Can you work these out from the drawing? Everything is in mm from the part's minimum corner. A direction names the side the tool comes from. Coordinates: 2 decimals unless noted, no trailing zeros. Loops run counter-clockwise (first coordinate to the right, second up) from the corner with the lowest first, then second, coordinate; pieces in that order, holes last.
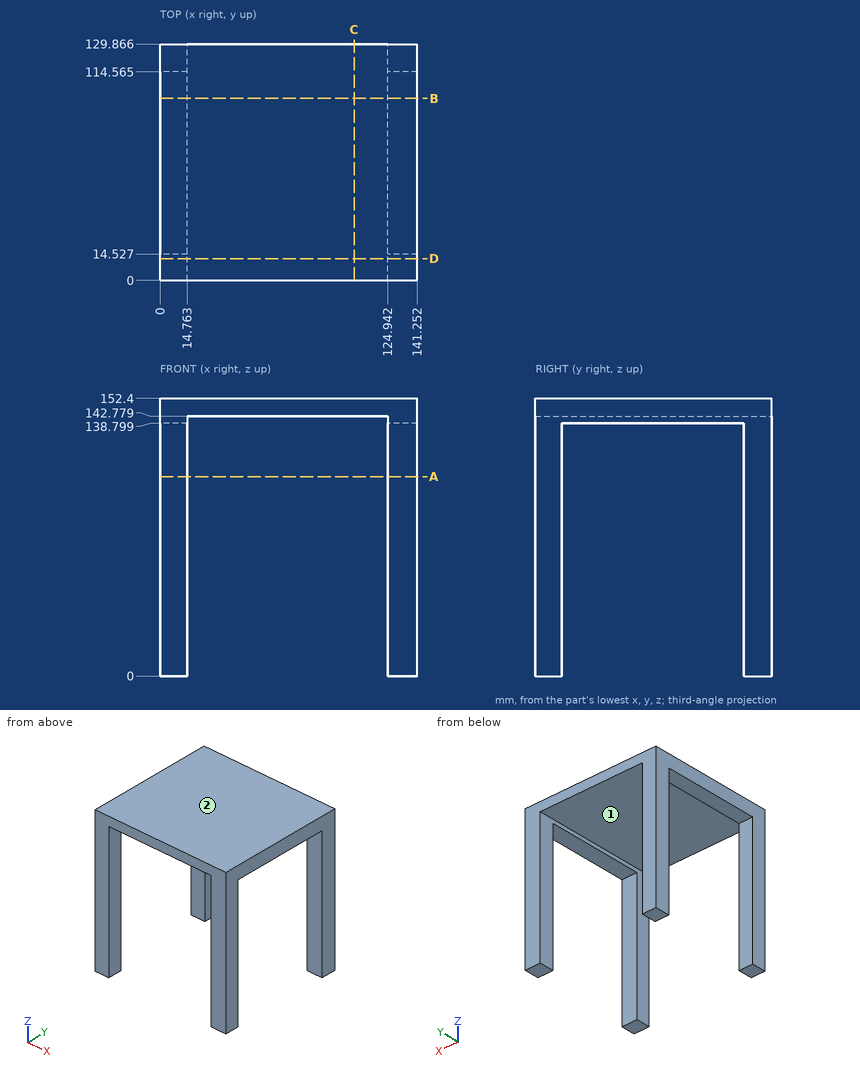
(1) Imagine slicing it at B-B, the plane y = 100. Write out the boundary of the cut face in (x, z), and give its area (3 significant figures).
Answers:
outline: (0, 138.8) - (14.76, 138.8) - (14.76, 142.78) - (124.94, 142.78) - (124.94, 138.8) - (141.25, 138.8) - (141.25, 152.4) - (0, 152.4) - close
area: 1,480 mm2
(2) Imagine slicing it at A-A, the plane z = 109.5. Write out the boundary of the cut face in (x, y) (1 decimal), and give its area (3 significant figures).
Answers:
outline: (0, 0) - (14.8, 0) - (14.8, 14.5) - (0, 14.5) - close; (0, 114.6) - (14.8, 114.6) - (14.8, 129.9) - (0, 129.9) - close; (124.9, 0) - (141.3, 0) - (141.3, 14.5) - (124.9, 14.5) - close; (124.9, 114.6) - (141.3, 114.6) - (141.3, 129.9) - (124.9, 129.9) - close
area: 927 mm2
(3) For pin 1 (3 mm diameter, centred on x = 78.5, y = 103, fed in from -Z); pin 2 (13 mm diameter, centred on x = 134.5, y = 58, fed in from -Z), each with a flat end and sliding along its axis, tell me the tip position at first contact or that it passes through.
Answers:
pin 1: stops at z = 142.78
pin 2: stops at z = 138.8
(4) Imagine slicing it at D-D, the plane y = 12. Write out the boundary of the cut face in (x, z).
Answers:
outline: (0, 0) - (14.76, 0) - (14.76, 142.78) - (124.94, 142.78) - (124.94, 0) - (141.25, 0) - (141.25, 152.4) - (0, 152.4) - close
(5) Which directions (+Z, -Z, +X, -X, +Y, -Y) give clear straight access to the entire face, cutting with the end or side of a thin tool? Please do the marked faces 1 and 2.
Answers:
face 1: -Z, +Y, -Y
face 2: +Z, +X, -X, +Y, -Y
(6) I need wall thicknesses on probe 1 along Y at (x, z) = (132, 28.5) (1 decimal); probe 2 along X at (y, z) = (124, 92.5); probe 3 along Z at (x, y) = (117, 66.5). Which ranges of each line are inside material? Lowest first, please.
Answers:
probe 1: y = 0 to 14.5, 114.6 to 129.9
probe 2: x = 0 to 14.76, 124.94 to 141.25
probe 3: z = 142.78 to 152.4
(7) Imagine slicing it at C-C, the plane x = 106.5. Write out the boundary of the cut face in (y, z).
Answers:
outline: (0, 142.78) - (129.87, 142.78) - (129.87, 152.4) - (0, 152.4) - close
